Here's the drawing with two shaded views (mm, measured from the low corner). I have some questions. A direction names the side the tool comes from. Coordinates: 2 decimals unless noted, no trailing zeros. Write each loop counter-clockwise with the first axis right and the second up, starting at its lowest first coordinate (ties: lowest second). Pieces come first, ordered by that corner, then holes.
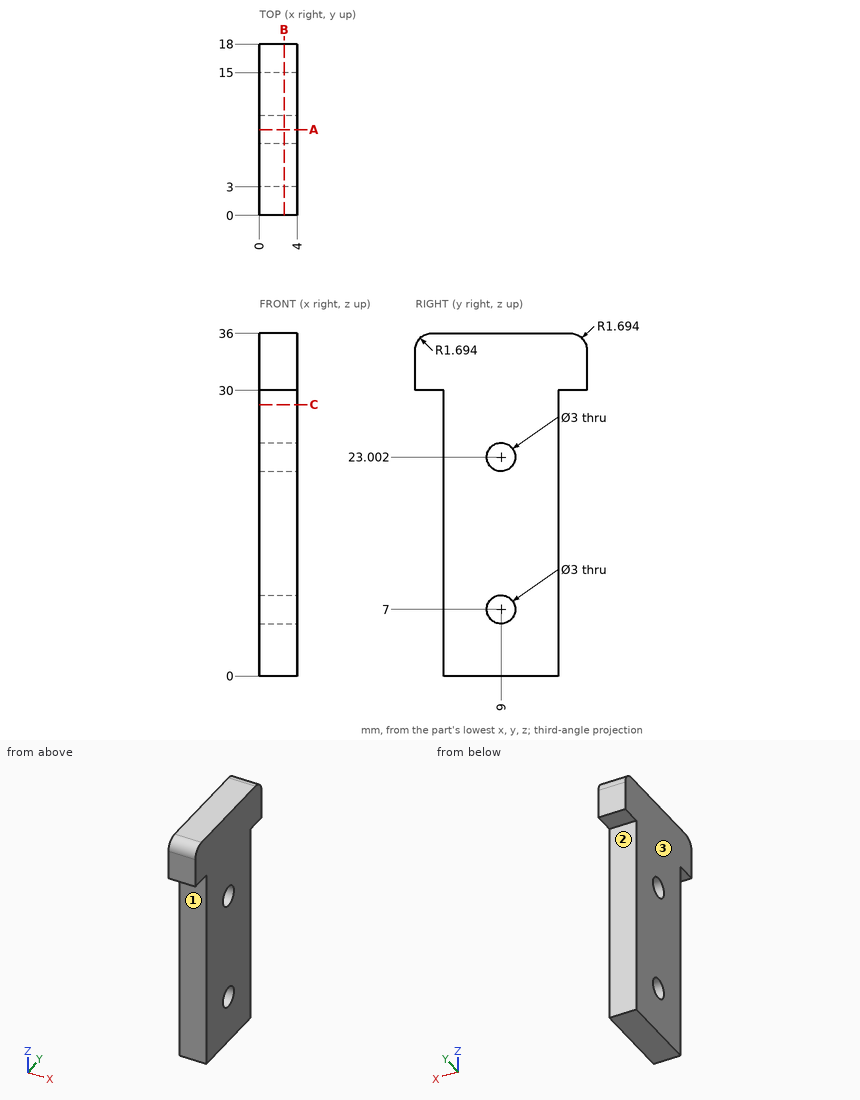
1. I want a section at B-B on x = 2.6. Please give me the cut outline in (y, z), plus the area to 3 significant figures.
Verdict:
outline: (0, 30) - (3, 30) - (3, 0) - (15, 0) - (15, 30) - (18, 30) - (18, 34.31) arc R1.69 ccw to (16.31, 36) - (1.69, 36) arc R1.69 ccw to (0, 34.31) - close; hole circle Ø3 at (9, 7); hole circle Ø3 at (9, 23)
area: 453 mm2
2. For pin 1 (2.5 mm diameter, centred on y = 9, z = 7, fed in from +X); pin 2 (1.5 mm diameter, centred on x = 2, z = 16, fed in from -Y); pin 3 (0.9 mm diameter, centred on x = 3, y = 16, fed in from -Z), each with a flat end and sliding along its axis, tell me the tip position at first contact or that it passes through.
Verdict:
pin 1: passes through
pin 2: stops at y = 3
pin 3: stops at z = 30
3. On a 3-axis mill with a long thin cutter (end or side, diameter ignored), from which of +Z, -Z, +X, -X, +Y, -Y can I reach the whole of each face in a straight line? I mean the marked faces 1, 2 and 3. Say none if no direction works.
Verdict:
face 1: -Z, +X, -X, -Y
face 2: -Z, +X, -X, +Y
face 3: +Z, -Z, -X, +Y, -Y
4. I want a section at A-A on y = 9. Please give me the cut outline in (x, z), plus the area to 3 significant figures.
Verdict:
outline: (0, 0) - (4, 0) - (4, 5.5) - (0, 5.5) - close; (0, 8.5) - (4, 8.5) - (4, 21.5) - (0, 21.5) - close; (0, 24.5) - (4, 24.5) - (4, 36) - (0, 36) - close
area: 120 mm2
5. Please list where these lines run through material, in increasing order: line 1 along Z through (x, y) = (3, 9); line 2 along Y through (x, z) = (2.75, 3); line 3 along Y through (x, z) = (2.2, 6).
Verdict:
line 1: z = 0 to 5.5, 8.5 to 21.5, 24.5 to 36
line 2: y = 3 to 15
line 3: y = 3 to 7.88, 10.12 to 15
6. I want a section at C-C on z = 28.5. Please give me the cut outline in (x, y), plus the area to 3 significant figures.
Verdict:
outline: (0, 3) - (4, 3) - (4, 15) - (0, 15) - close
area: 48.0 mm2
